from build123d import *

# Parameters (mm, degrees)
BOSS_EXTRUDE1_DEPTH      = 101.6
FILLET1_R                = 2.54
SKETCH11_R               = 8.41375
CUT_EXTRUDE8_DEPTH       = 1
CUT_EXTRUDE8_DEPTH_BACK  = 44.994090512
SKETCH12_R               = 8.41375
CUT_EXTRUDE9_DEPTH       = 18.348522628
CUT_EXTRUDE9_DEPTH_BACK  = 62.34261314
SKETCH13_R               = 8.41375
CUT_EXTRUDE10_DEPTH      = 18.348522628
CUT_EXTRUDE10_DEPTH_BACK = 62.34261314


with BuildPart() as part:
    # Sketch2 → Boss-Extrude1 (new body)
    with BuildSketch(Plane(origin=(0, 0, 0), x_dir=(1, 0, 0), z_dir=(0, 1, 0))):
        with BuildLine():
            Line((-23.65375, 3.024593723), (-21.733825791, 6.35))
            Line((-21.733825791, 6.35), (-32.732348419, 6.35))
            Line((-32.732348419, 6.35), (-32.732348419, -6.35))
            Line((-32.732348419, -6.35), (-21.733825791, -6.35))
            Line((-21.733825791, -6.35), (-23.65375, -3.024593723))
            ThreePointArc((-23.65375, -3.024593723), (-28.8925, 0), (-23.65375, 3.024593723))
        make_face()
        with BuildLine():
            Line((32.732348419, 6.35), (21.733825791, 6.35))
            Line((21.733825791, 6.35), (23.65375, 3.024593723))
            ThreePointArc((23.65375, 3.024593723), (27.14625, 3.024593723), (28.8925, 0))
            ThreePointArc((28.8925, 0), (27.14625, -3.024593723), (23.65375, -3.024593723))
            Line((23.65375, -3.024593723), (21.733825791, -6.35))
            Line((21.733825791, -6.35), (32.732348419, -6.35))
            Line((32.732348419, -6.35), (32.732348419, 6.35))
        make_face()
        Polygon((12.7, 21.997045256), (-12.7, 21.997045256), (-21.733825791, 6.35), (-18.067651581, 6.35), (-10.866912895, 18.822045256), (10.866912895, 18.822045256), (18.067651581, 6.35), (21.733825791, 6.35), align=None)
        Polygon((-10.866912895, -18.822045256), (-18.067651581, -6.35), (-21.733825791, -6.35), (-12.7, -21.997045256), (12.7, -21.997045256), (21.733825791, -6.35), (18.067651581, -6.35), (10.866912895, -18.822045256), align=None)
        with BuildLine():
            Line((-18.067651581, 6.35), (-21.733825791, 6.35))
            Line((-21.733825791, 6.35), (-23.65375, 3.024593723))
            ThreePointArc((-23.65375, 3.024593723), (-22.375406277, 1.74625), (-21.9075, 0))
            ThreePointArc((-21.9075, 0), (-22.375406277, -1.74625), (-23.65375, -3.024593723))
            Line((-23.65375, -3.024593723), (-21.733825791, -6.35))
            Line((-21.733825791, -6.35), (-18.067651581, -6.35))
            Line((-18.067651581, -6.35), (-21.733825791, 0))
            Line((-21.733825791, 0), (-18.067651581, 6.35))
        make_face()
        Polygon((-18.067651581, -6.35), (-18.067651581, 6.35), (-21.733825791, 0), align=None)
        with BuildLine():
            Line((23.65375, 3.024593723), (21.733825791, 6.35))
            Line((21.733825791, 6.35), (18.067651581, 6.35))
            Line((18.067651581, 6.35), (21.733825791, 0))
            Line((21.733825791, 0), (18.067651581, -6.35))
            Line((18.067651581, -6.35), (21.733825791, -6.35))
            Line((21.733825791, -6.35), (23.65375, -3.024593723))
            ThreePointArc((23.65375, -3.024593723), (21.9075, 0), (23.65375, 3.024593723))
        make_face()
        Polygon((21.733825791, 0), (18.067651581, 6.35), (18.067651581, -6.35), align=None)
    extrude(amount=BOSS_EXTRUDE1_DEPTH)

    # Fillet1
    fillet1_edges = [part.edges().sort_by_distance(p)[0] for p in [
        (21.733825791, 50.8, -6.35),
        (32.732348419, 50.8, -6.35),
        (32.732348419, 50.8, 6.35),
        (21.733825791, 50.8, 6.35),
        (-21.733825791, 50.8, 6.35),
        (-32.732348419, 50.8, 6.35),
        (-32.732348419, 50.8, -6.35),
        (-21.733825791, 50.8, -6.35),
    ]]
    fillet(fillet1_edges, radius=FILLET1_R)

    # Sketch11 → Cut-Extrude8 (cut, two sides)
    with BuildSketch(Plane(origin=(0, 0, -21.997045256), x_dir=(-1, 0, 0), z_dir=(0, 0, -1))) as cut_extrude8_sk:
        with Locations((0, 76.2)):
            Circle(SKETCH11_R)
    extrude(amount=CUT_EXTRUDE8_DEPTH, mode=Mode.SUBTRACT)
    extrude(cut_extrude8_sk.sketch, amount=-CUT_EXTRUDE8_DEPTH_BACK, mode=Mode.SUBTRACT)

    # Sketch12 → Cut-Extrude9 (cut, two sides)
    with BuildSketch(Plane(origin=(-19.05, 0, -10.998522628), x_dir=(-0.5, 0, 0.866025404), z_dir=(-0.866025404, 0, -0.5))) as cut_extrude9_sk:
        with Locations((0, 50.8)):
            Circle(SKETCH12_R)
    extrude(amount=CUT_EXTRUDE9_DEPTH, mode=Mode.SUBTRACT)
    extrude(cut_extrude9_sk.sketch, amount=-CUT_EXTRUDE9_DEPTH_BACK, mode=Mode.SUBTRACT)

    # Sketch13 → Cut-Extrude10 (cut, two sides)
    with BuildSketch(Plane(origin=(19.05, 0, -10.998522628), x_dir=(-0.5, 0, -0.866025404), z_dir=(0.866025404, 0, -0.5))) as cut_extrude10_sk:
        with Locations((0, 25.4)):
            Circle(SKETCH13_R)
    extrude(amount=CUT_EXTRUDE10_DEPTH, mode=Mode.SUBTRACT)
    extrude(cut_extrude10_sk.sketch, amount=-CUT_EXTRUDE10_DEPTH_BACK, mode=Mode.SUBTRACT)


solid = part.part
Work out the finished part from the listing and answer in its coordinate system (mm). A direction names the side the tool comes from. Give positions to 0.01 mm unless a question says otherwise; leave off trailing zeros. Write each loop counter-clockwise with the first axis right and the second up, starting at its lowest first coordinate (ties: lowest second). Pieces come first, ordered by that corner, then holes. Notation, with made-up numbers: M 0,22.25 L 59,22.25 A28 cw 59,59.25 Z; hole C -13,6 d4. An arc over 180 degrees is marked long. Answer as CSV lines item,"result".
Q1. A cutting plane is placed at B-B on y = 92. Count the separate pieces of the cut face and the enclosed holes in it, plus the area to 3 significant figures.
A:
separate pieces,"1"
enclosed holes,"3"
area,"648 mm²"
Q2. Given P1, Ø7.5, axis at x = -25.5, y = 59, coming from the +Z side; P2, Ø8, axis at x = -24, z = 1, coming from the -Y side; P3, Ø4, axis at x = 24, y = 50, coming from the -Z side; P4, Ø2, axis at x = 26, y = 38.5, coming from the -Z side, each flat-ended and moving along its own axis, determine where each tip first touches the part or whether it passes through.
A:
P1,"stops at z = 6.8"
P2,"stops at y = 0"
P3,"stops at z = -6.65"
P4,"stops at z = -6.35"
Q3. A cutting plane is placed at A-A on x = 0. Write down the section's boundary in (y, z), plus the area to 3 significant figures.
A:
outline,"M 0,-22 L 67.79,-22 L 67.79,-18.82 L 0,-18.82 Z; M 0,18.82 L 67.79,18.82 L 67.79,22 L 0,22 Z; M 84.61,-22 L 101.6,-22 L 101.6,-18.82 L 84.61,-18.82 Z; M 84.61,18.82 L 101.6,18.82 L 101.6,22 L 84.61,22 Z"
area,"538 mm²"
Q4. Find the intervals of material crossed by probe 1 along Y at (x, z) = (0, -20.25); probe 2 along X at (y, z) = (82.5, 4); probe 3 along Z at (x, y) = (-7, 9.5), in increasing order. Write a range as [from, to].
A:
probe 1,"y = [0, 67.79], [84.61, 101.6]"
probe 2,"x = [-32.73, -18.07], [18.07, 32.73]"
probe 3,"z = [-22, -18.82], [18.82, 22]"
Q5. A tool of negligible diameter and unlimited length cuts with its end or side. For faces 1 (the flat face through (16.908, 50.089, -14.708)), 2 (the flat face through (14.4, 50.1, -12.7)), 3 (the flat face through (-28, 50, -6.35)), from which of +Z, -Z, +X, -X, +Y, -Y can it reach the whole face along a straight path? Write none if from no direction.
A:
face 1,"-Z, +X, +Y, -Y"
face 2,"+Y, -Y"
face 3,"-Z, -X, +Y, -Y"
Q6. The mould has two halves that part along Z. Classify faces 4 (the flat face through (-20, 0, 0)), 5 (the flat face through (0, 50, -18.822)), 6 (the cylindrical face through (31.969, 51.511, 5.626)), 7 (the cylindrical face through (-31.969, 51.511, -5.626)): +Z half, -Z half, draft (parallel to the pull), parting line (faces both ways), or undercut.
A:
face 4,"draft"
face 5,"undercut"
face 6,"+Z half"
face 7,"-Z half"
